Here's how the part is built. I have some questions about the finished solid (model axes, mm). Face numbers are marked on the shaded views. A direction names the side the tool comes from. Give positions to 0.01 mm unless a question says otherwise; leave off trailing zeros. Loops run counter-clockwise (first coordinate to the right, second up) from the corner with the lowest first, then second, coordinate; pieces in that order, holes last.
Q1. Will these pins go through, and if not, where does the flat tip stop? P1, Ø8, axis at x = 6.5, z = -8, coming from the -Y side; P2, Ø12, axis at x = 14, y = -27.5, coming from the -Z side.
Q2. For the marked faces 4 and 5, which set-ups out of +Z, -Z, +X, -X, +Y, -Y let a thin tool reach every point of the face, with its end or its side?
Q3. If we section it at D-D (x = 7): Please give me the cut outline in (y, z), plus the area to 3 significant figures.
Q4. I need wall thicknesses on line 1 (X direction, y = -132.5, z = -11); line 2 (Z direction, x = 23, y = -41); line 3 (Y direction, x = -14, z = -27). Which ranges of each line are inside material? Lowest first, please.
Q5. If we section it at B-B (y = -88): Please give me the cut outline in (x, z), plus the area to 3 significant figures.
Q6. We'd pull the mould along X, two halves only. Please class the marked faces 1, 2 and 3: +X half, -X half, draft (parallel to the pull), parting line (faces both ways), or undercut.
Q7. If we section it at C-C (x = -27): Please give me the cut outline in (y, z).
Q8. If we section it at A-A (z = 2.5): Please give me the cut outline in (x, y).
from build123d import *

# Parameters (mm, degrees)
F0_W     = 94
F0_H     = 60
F1_DEPTH = 150
F2_T     = -1
F4_DEPTH = 60.001


with BuildPart() as f1:
    # F0 (on Front) → F1 (new body)
    with BuildSketch(Plane.XZ):
        Rectangle(F0_W, F0_H)
    extrude(amount=F1_DEPTH)

    # F2
    f2_openings = [f1.faces().sort_by_distance(p)[0] for p in [
        (0, -150, 0),
        (0, -75, -30),
    ]]
    offset(amount=F2_T, openings=f2_openings)

    # F3 (on face) → F4 (cut, through all)
    with BuildSketch(Plane.XY.offset(30)):
        with BuildLine():
            Line((47, -150), (47, -135))
            ThreePointArc((47, -135), (0, -142.553519), (-47, -135))
            Line((-47, -135), (-47, -150))
            Line((-47, -150), (47, -150))
        make_face()
    extrude(amount=-F4_DEPTH, mode=Mode.SUBTRACT)


solid = f1.part
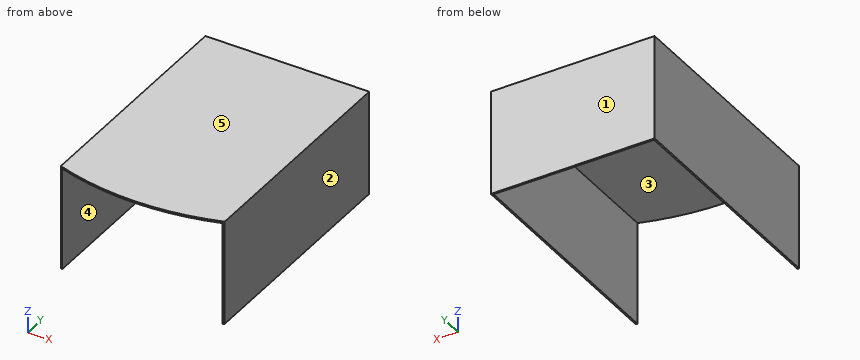
Check sheet entries:
1. P1: stops at y = -1
1. P2: stops at z = 29
2. face 4: -Z, -Y
2. face 5: +Z, +X, -X, +Y, -Y
3. outline: (-142.39, 29) - (-1, 29) - (-1, -30) - (0, -30) - (0, 30) - (-142.39, 30) - close
3. area: 201 mm2
4. line 1: x = -47 to -46, 46 to 47
4. line 2: z = 29 to 30
4. line 3: y = -1 to 0
5. outline: (-47, -30) - (-46, -30) - (-46, 29) - (46, 29) - (46, -30) - (47, -30) - (47, 30) - (-47, 30) - close
5. area: 212 mm2
6. face 1: draft
6. face 2: +X half
6. face 3: undercut
7. outline: (-140.1, 29) - (-1, 29) - (-1, -30) - (0, -30) - (0, 30) - (-140.1, 30) - close
8. outline: (-47, -135) arc R150 ccw to (-46, -135.33) - (-46, -1) - (46, -1) - (46, -135.33) arc R150 ccw to (47, -135) - (47, 0) - (-47, 0) - close
